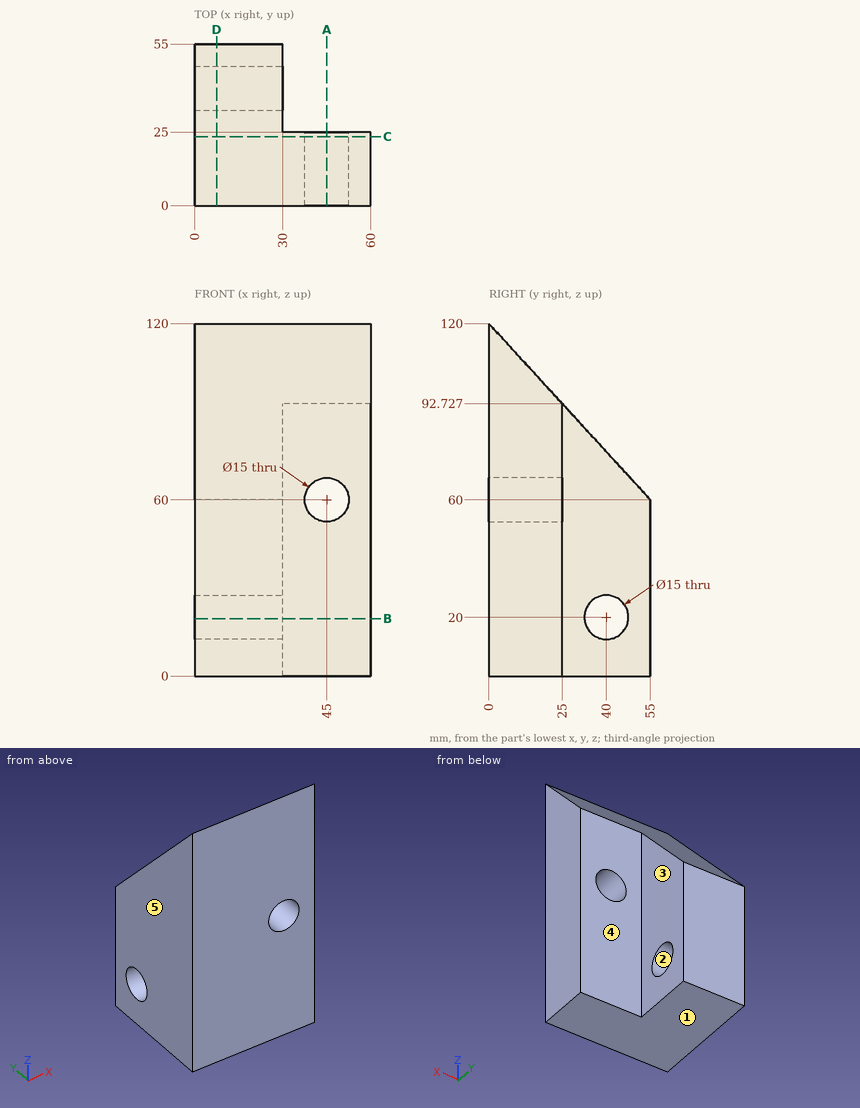
The drawing under review shows one solid part. Ordinate dimensions are in mm from its lowest x, y, z. A direction names the side the tool comes from. Coordinates: 2 decimals unless noted, no trailing zeros. Write each loop counter-clockwise with the first axis right and the second up, starting at its lowest first coordinate (ties: lowest second). Pieces come first, ordered by that corner, then holes. Notation, with made-up numbers: (85.5, 79) -> (114.5, 79) arc R25 ccw to (114.5, 110) -> close; hole circle Ø4 at (83.5, -15.75). An arc over 180 degrees is marked (long way). One line per item, written item: value. Start each with the question number.
Q1. Add section D-D, the plane x = 7.5. Give the boundary of the cut face in (y, z), then the cut area to 3 significant figures.
Q2. Add section A-A, the plane x = 45. Give the boundary of the cut face in (y, z), then the cut area to 3 significant figures.
Q3. Add section B-B, the plane z = 19.5. Give the boundary of the cut face in (x, y).
Q4. Clearance check with flat-ended pins moving along their axes: P1, Ø1, axis at y = 16, z = 45.5, coming from the -X side; P2, Ø10, axis at y = 33, z = 42, coming from the +X side; P3, Ø9, axis at x = 46, z = 49.5, coming from the +Y side; P4, Ø3, axis at x = 23, y = 16, coming from the +Z side. State where each tip first meets the part, or that it passes through.
Q5. To check wall thickness, follow probe 1 along Y at (x, z) = (15, 20); probe 2 along X at (y, z) = (17, 60); probe 3 along X at (y, z) = (29, 17). State the ranges of each line that lie inside material, in increasing order.
Q6. For the marked faces 4 and 5, list the 3-axis set-ups (+Z, -Z, +X, -X, +Y, -Y) from which the entire face can be reached by the end or side of a thin tool; tool diameter is ignored.
Q7. The part is to be moulded in two halves that separate along Z. For the marked faces 1, 2 and 3, say which applies: +Z half, -Z half, draft (parallel to the pull), parting line (faces both ways), or undercut.
Q8. Add section C-C, the plane y = 23.5. Give the boundary of the cut face in (x, z).
Response:
1. outline: (0, 0) -> (55, 0) -> (55, 60) -> (0, 120) -> close; hole circle Ø15 at (40, 20)
1. area: 4,770 mm²
2. outline: (0, 0) -> (25, 0) -> (25, 52.5) -> (0, 52.5) -> close; (0, 67.5) -> (25, 67.5) -> (25, 92.73) -> (0, 120) -> close
2. area: 2,280 mm²
3. outline: (0, 0) -> (60, 0) -> (60, 25) -> (30, 25) -> (30, 32.52) -> (0, 32.52) -> close; (0, 47.48) -> (30, 47.48) -> (30, 55) -> (0, 55) -> close
4. P1: x = 0
4. P2: x = 30
4. P3: y = 25
4. P4: z = 104.18
5. probe 1: 0 to 32.5, 47.5 to 55
5. probe 2: 0 to 37.5, 52.5 to 60
5. probe 3: 0 to 30
6. face 4: +Z, -Z, +X, +Y
6. face 5: +Z, -Z, -X, +Y, -Y
7. face 1: -Z half
7. face 2: undercut
7. face 3: draft
8. outline: (0, 0) -> (60, 0) -> (60, 94.36) -> (0, 94.36) -> close; hole circle Ø15 at (45, 60)
